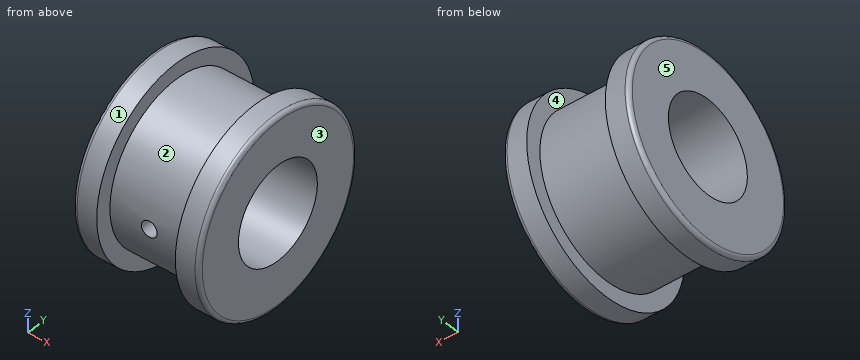
```python
from build123d import *

# Parameters (mm, degrees)
SKETCH_2_R               = 12
EXTRUDE_1_DEPTH          = 8
SKETCH_3_R               = 12
SKETCH_3_R_2             = 10
CUT_EXTRUDE_1_DEPTH      = 5
SKETCH_4_R               = 6
CUT_EXTRUDE_2_DEPTH      = 9
CUT_EXTRUDE_2_DEPTH_BACK = 9
FILLET_1_R               = 0.5
SKETCH_5_R               = 1
CUT_EXTRUDE_3_DEPTH      = 10


with BuildPart() as part:
    # 草图2 → 凸台-拉伸1 (new body, symmetric)
    with BuildSketch(Plane(origin=(0, 0, 0), x_dir=(0, 0, -1), z_dir=(1, 0, 0))):
        Circle(SKETCH_2_R)
    extrude(amount=EXTRUDE_1_DEPTH, both=True)

    # 草图3 → 切除-拉伸1 (cut, symmetric)
    with BuildSketch(Plane(origin=(0, 0, 0), x_dir=(0, 0, -1), z_dir=(1, 0, 0))):
        Circle(SKETCH_3_R)
        Circle(SKETCH_3_R_2, mode=Mode.SUBTRACT)
    extrude(amount=CUT_EXTRUDE_1_DEPTH, both=True, mode=Mode.SUBTRACT)

    # 草图4 → 切除-拉伸2 (cut, two sides)
    with BuildSketch(Plane(origin=(0, 0, 0), x_dir=(0, 0, -1), z_dir=(1, 0, 0))) as cut_extrude_2_sk:
        Circle(SKETCH_4_R)
    extrude(amount=CUT_EXTRUDE_2_DEPTH, mode=Mode.SUBTRACT)
    extrude(cut_extrude_2_sk.sketch, amount=-CUT_EXTRUDE_2_DEPTH_BACK, mode=Mode.SUBTRACT)

    # 圆角1
    fillet_1_edges = [part.edges().sort_by_distance(p)[0] for p in [
        (-8, 0, 12),
        (8, 0, 12),
    ]]
    fillet(fillet_1_edges, radius=FILLET_1_R)

    # 草图5 → 切除-拉伸3 (cut)
    with BuildSketch(Plane(origin=(0, 0, 0), x_dir=(1, 0, 0), z_dir=(0, 1, 0))):
        Circle(SKETCH_5_R)
    extrude(amount=-CUT_EXTRUDE_3_DEPTH, mode=Mode.SUBTRACT)


solid = part.part
```
Here's how the part is built. I have some questions about the finished solid (model axes, mm). Face numbers are marked on the shaded views. A direction names the side the tool comes from. Round coordinates to 2 decimals unless told otherwise and drop trailing zeros. Order: outer loops, then holes, each group sorted by start corner. A loop starts at its lowest first (then second) coordinate and runs counter-clockwise, first axis right, second up. Notation, with made-up numbers: (13.25, 35) -> (56.25, 35) arc R22 cw to (56.25, 74) -> close; hole circle Ø10 at (13, 19.5). An arc over 180 degrees is marked (long way). Use a Markdown table: item, result. Add a question column.
(1) If we mould it in two halves opening along X, with no side actions, what happens to the marked faces 3, 4 and 5? For each: released by +X, released by -X, zero draft, split by the parting line, or undercut.
(2) For pin 1 Ø1.5 at (x, z) = (5.5, -9.5) entering from +Y; pin 2 Ø1.2 at (x, z) = (0, 0) entering from +Y; pin 3 Ø2 at (x, y) = (-1.5, -2.5) entering from +Z; pin 4 Ø6 at (y, z) = (3.5, -2) entering from +X, each with a flat end and sliding along its axis, tell me the tip position at first contact or that it passes through.
(3) Suppose I cut it at A-A, the plane y = 0. Please give me the cut outline in (x, z), and give its area (3 significant figures).
(4) Suppose I cut it at D-D, the plane x = -5.5. Please give me the cut outline in (y, z).
(5) For the marked faces 1 and 2, which set-ups out of +Z, -Z, +X, -X, +Y, -Y let a thin tool reach every point of the face, with its end or its side?
(6) Suppose I cut it at B-B, the plane z = 0. Please give me the cut outline in (x, y), and give its area (3 significant figures).
(7) Suppose I cut it at C-C, the plane x = -3.25. Please give me the cut outline in (y, z).
(8) I need wall thicknesses on line 1 along Y through (x, z) = (-1.25, -0.25); line 2 along X through (y, z) = (-4, -9.5); line 3 along X through (y, z) = (-8.65, 0). Which ranges of each line are inside material? Lowest first, please.
Verdict:
| question | item | result |
|---|---|---|
| 1 | face 3 | released by +X |
| 1 | face 4 | undercut |
| 1 | face 5 | released by -X |
| 2 | pin 1 | y = 8.21 |
| 2 | pin 2 | y = 10 |
| 2 | pin 3 | z = 9.89 |
| 2 | pin 4 | x = 8 |
| 3 | outline | (-8, -11.5) arc R0.5 ccw to (-7.5, -12) -> (-5, -12) -> (-5, -10) -> (5, -10) -> (5, -12) -> (7.5, -12) arc R0.5 ccw to (8, -11.5) -> (8, -6) -> (-8, -6) -> close; (-8, 6) -> (8, 6) -> (8, 11.5) arc R0.5 ccw to (7.5, 12) -> (5, 12) -> (5, 10) -> (-5, 10) -> (-5, 12) -> (-7.5, 12) arc R0.5 ccw to (-8, 11.5) -> close |
| 3 | area | 152 mm2 |
| 4 | outline | circle Ø24 at (0, 0); hole circle Ø12 at (0, 0) |
| 5 | face 1 | +X, -X |
| 5 | face 2 | none |
| 6 | outline | (-8, -11.5) arc R0.5 ccw to (-7.5, -12) -> (-5, -12) -> (-5, -10) -> (-1, -10) -> (-1, -6) -> (-8, -6) -> close; (-8, 6) -> (8, 6) -> (8, 11.5) arc R0.5 ccw to (7.5, 12) -> (5, 12) -> (5, 10) -> (-5, 10) -> (-5, 12) -> (-7.5, 12) arc R0.5 ccw to (-8, 11.5) -> close; (1, -10) -> (5, -10) -> (5, -12) -> (7.5, -12) arc R0.5 ccw to (8, -11.5) -> (8, -6) -> (1, -6) -> close |
| 6 | area | 144 mm2 |
| 7 | outline | circle Ø20 at (0, 0); hole circle Ø12 at (0, 0) |
| 8 | line 1 | -10 to -5.99, 5.99 to 10 |
| 8 | line 2 | -8 to -5, 5 to 8 |
| 8 | line 3 | -8 to -1, 1 to 8 |
